from build123d import *

# Parameters (mm, degrees)
PAD_DEPTH       = 5
SKETCH002_R     = 15
SKETCH003_R     = 11
POCKET_DEPTH    = 7.2
SKETCH004_R     = 5
POCKET001_DEPTH = 1.801
SKETCH005_R     = 2.6
POCKET002_DEPTH = 5.001
CHAMFER_SIZE    = 2
CHAMFER001_SIZE = 4
CHAMFER002_SIZE = 2


with BuildPart() as part:
    # Sketch → Pad (new body)
    with BuildSketch(Plane.XY):
        with BuildLine():
            Line((-21, 20), (-21, 0))
            Line((-21, 0), (21, 0))
            Line((21, 0), (21, 20))
            Line((14.492167, 44.370025), (21, 20))
            ThreePointArc((14.492167, 44.370025), (0, 55.5), (-14.492167, 44.370025))
            Line((-14.492167, 44.370025), (-21, 20))
        make_face()
    extrude(amount=PAD_DEPTH)

    # Sketch001 (on Face8 of Pad) → AdditiveLoft section 0
    with BuildSketch(Plane.XY.offset(5)):
        with BuildLine():
            Line((-21, 20), (21, 20))
            Line((21, 20), (14.492167, 44.370025))
            ThreePointArc((14.492167, 44.370025), (0, 55.5), (-14.492167, 44.370025))
            Line((-14.492167, 44.370025), (-21, 20))
        make_face()
    # Sketch002 (on DatumPlane) → AdditiveLoft section 1
    with BuildSketch(Plane.XY.offset(9)):
        with Locations((0, 40.5)):
            Circle(SKETCH002_R)
    loft()

    # Sketch003 (on Face12 of AdditiveLoft) → Pocket (cut)
    with BuildSketch(Plane.XY.offset(9)):
        with Locations((0, 40.5)):
            Circle(SKETCH003_R)
    extrude(amount=-POCKET_DEPTH, mode=Mode.SUBTRACT)

    # Sketch004 (on Face16 of Pocket) → Pocket001 (cut, through all)
    with BuildSketch(Plane.XY.offset(1.8)):
        with Locations((0, 40.5)):
            Circle(SKETCH004_R)
    extrude(amount=-POCKET001_DEPTH, mode=Mode.SUBTRACT)

    # Sketch005 (on Face14 of Pocket001) → Pocket002 (cut, through all)
    with BuildSketch(Plane.XY.offset(5)):
        with Locations((-11, 10)):
            Circle(SKETCH005_R)
        with Locations((11, 10)):
            Circle(SKETCH005_R)
    extrude(amount=-POCKET002_DEPTH, mode=Mode.SUBTRACT)

    # Chamfer
    chamfer_edges = [part.edges().sort_by_distance(p)[0] for p in [
        (-11, 40.5, 9),
    ]]
    chamfer(chamfer_edges, length=CHAMFER_SIZE)

    # Chamfer001
    chamfer001_edges = [part.edges().sort_by_distance(p)[0] for p in [
        (21, 0, 2.5),
        (-21, 0, 2.5),
    ]]
    chamfer(chamfer001_edges, length=CHAMFER001_SIZE)

    # Chamfer002
    chamfer002_edges = [part.edges().sort_by_distance(p)[0] for p in [
        (-19, 2, 0),
        (0, 0, 0),
        (19, 2, 0),
        (21, 12, 0),
        (17.746084, 32.185012, 0),
        (0, 55.5, 0),
        (-17.746084, 32.185012, 0),
        (-21, 12, 0),
    ]]
    chamfer(chamfer002_edges, length=CHAMFER002_SIZE)


solid = part.part
Can you work these out from the model? Positions are in its coordinate system, mm. A direction names the side the tool comes from. Round coordinates to 2 decimals unless told otherwise and drop trailing zeros. Order: outer loops, then holes, each group sorted by start corner. A loop starts at its lowest first (then second) coordinate and runs counter-clockwise, first axis right, second up. Notation, with made-up numbers: M -33.75,88.5 L -24.75,88.5 A13 cw -24.75,98.5 Z; hole C 22.25,49.5 d7. An arc over 180 degrees is marked long. Use a Markdown table: item, result.
1) Imagine slicing it at A-A (z = 3). List the corners of the cut face in (x, y) for me, then the cut area to 3 significant figures.
Geometry says:
| item | result |
|---|---|
| outline | M -21,4 L -17,0 L 17,0 L 21,4 L 21,20 L 14.49,44.37 A15 ccw -14.49,44.37 L -21,20 Z; hole C -11,10 d5.2; hole C 0,40.5 d22; hole C 11,10 d5.2 |
| area | 1,500 mm² |
2) On a 3-axis mill with a long thin cutter (end or side, diameter ignored), from which of +Z, -Z, +X, -X, +Y, -Y can I reach the whole of each face in a straight line? I mean faces 5 (the face through (-1.432, 51.406, 4.436)), 6 (the face through (19, 2, 3)), 7 (the face through (0, 10, 5)). Say none if no direction works.
Geometry says:
| item | result |
|---|---|
| face 5 | +Z |
| face 6 | +Z, -Z, +X, -Y |
| face 7 | +Z, +X, -X, -Y |
3) Imagine slicing it at B-B (y = 15). List the corners of the cut face in (x, z) for me, then the cut area to 3 significant figures.
Geometry says:
| item | result |
|---|---|
| outline | M -21,2 L -19,0 L 19,0 L 21,2 L 21,5 L -21,5 Z |
| area | 206 mm² |
4) If we mould it in two halves opening along Y, with no side actions, what happens to faces 1 (the face through (17.7, 32.36, 3.48)), 2 (the face through (2.3, 35.8, 1.8)), 3 (the face through (-0.651, 45.457, 0.913)), 4 (the face through (18.311, 2.745, 0.986))? For each: +Y half, -Y half, draft (parallel to the pull), parting line (faces both ways), or undercut.
Geometry says:
| item | result |
|---|---|
| face 1 | +Y half |
| face 2 | undercut |
| face 3 | undercut |
| face 4 | -Y half |
5) If I drill on line 1 along Y through (x, z) = (0, 2.95); line 2 along Y through (x, z) = (2.5, 7); line 3 along Z through (x, y) = (19, 17), over which ranges is the centre line in solid material (lowest first)?
Geometry says:
| item | result |
|---|---|
| line 1 | y = 0 to 29.5, 51.5 to 55.5 |
| line 2 | y = 22.82 to 29.79, 51.21 to 55.28 |
| line 3 | z = 0 to 5 |
6) I'm going to push flat-ended pins straight in: P1, Ø13, axis at x = 0, y = 40.5, coming from the +Z side; P2, Ø3, axis at y = 43.5, z = 5.5, coming from the -X side; P3, Ø6, axis at x = 7, y = 14, coming from the +Z side; P4, Ø9, axis at x = 0, y = 40.5, coming from the -Z side. Where does each tip first touch, or does it pass through?
Geometry says:
| item | result |
|---|---|
| P1 | stops at z = 1.8 |
| P2 | stops at x = -15.1 |
| P3 | stops at z = 5 |
| P4 | passes through |
